```python
from build123d import *

# Parameters (mm, degrees)
SKETCH1_R           = 50
BOSS_EXTRUDE1_DEPTH = 150
SKETCH2_R           = 50
BOSS_EXTRUDE2_DEPTH = 150


with BuildPart() as part:
    # Sketch1 → Boss-Extrude1 (new, symmetric)
    with BuildSketch(Plane(origin=(0, 0, 0), x_dir=(1, 0, 0), z_dir=(0, 1, 0))):
        with Locations(Location((0, 0, 0), (0, 0, 270))):
            Circle(SKETCH1_R)
    extrude(amount=BOSS_EXTRUDE1_DEPTH, both=True)

    # Sketch2 → Boss-Extrude2 (add, symmetric)
    with BuildSketch(Plane(origin=(0, 0, 0), x_dir=(0, 0, -1), z_dir=(1, 0, 0))):
        Circle(SKETCH2_R)
    extrude(amount=BOSS_EXTRUDE2_DEPTH, both=True)


solid = part.part
```
Check sheet for the modelled part. Datum: model origin and axes. Units: mm. A direction names the side the tool comes from. Give positions to 0.01 mm unless a question says otherwise; leave off trailing zeros. Order: outer loops, then holes, each group sorted by start corner. A loop starts at its lowest first (then second) coordinate and runs counter-clockwise, first axis right, second up. Notation, with made-up numbers: M -37.5,88.25 L 5.5,88.25 A8 cw 5.5,93.25 Z; hole C 89,-9 d7. An arc over 180 degrees is marked long. Answer in a Markdown table with one row per item.
1) Cross-section at D-D, the plane z = -21. Enter the section's corners in (x, y), plus the area to 3 significant figures.
Filled sheet:
| item | result |
|---|---|
| outline | M -150,-45.38 L -45.38,-45.38 L -45.38,-150 L 45.38,-150 L 45.38,-45.38 L 150,-45.38 L 150,45.38 L 45.38,45.38 L 45.38,150 L -45.38,150 L -45.38,45.38 L -150,45.38 Z |
| area | 46,200 mm2 |
2) Access from +Z, -Z, +X, -X, +Y, -Y to the whole of each face (thin tool, end or side, straight path). Record for faces 1 (the cylindrical face through (49.575, 92.717, -6.509)), 2 (the cylindrical face through (2.2, -90.62, -49.95)), 3 (the cylindrical face through (92.717, 49.575, 6.509)).
Filled sheet:
| item | result |
|---|---|
| face 1 | +Y |
| face 2 | -Y |
| face 3 | +X |
3) Thickness scan on L1, parallel to Z at x = 119, y = -1; L2, parallel to X at y = 96, z = 1.5; L3, parallel to X at y = -59.5, z = -6. Record the ranges inside material, lowest first. Write a range as [from, to].
Filled sheet:
| item | result |
|---|---|
| L1 | z = [-49.99, 49.99] |
| L2 | x = [-49.98, 49.98] |
| L3 | x = [-49.64, 49.64] |
4) Cross-section at C-C, the plane x = 15. Enter the section's corners in (y, z).
Filled sheet:
| item | result |
|---|---|
| outline | M -150,-47.7 L -15,-47.7 A50 ccw 15,-47.7 L 150,-47.7 L 150,47.7 L 15,47.7 A50 ccw -15,47.7 L -150,47.7 Z |
5) Gauge pin test, flat ends, axial feed: P1, Ø8, axis at x = 31, y = -32.5, coming from the +Z side; P2, Ø2, axis at x = -20, y = 19.5, coming from the -Z side; P3, Ø1.5, axis at x = 100, z = -36, coming from the -Y side. Record the tip position at first contact, or that the pin passes through.
Filled sheet:
| item | result |
|---|---|
| P1 | stops at z = 42.08 |
| P2 | stops at z = -46.45 |
| P3 | stops at y = -35.46 |
6) Cross-section at A-A, the plane z = 0. Enter the section's corners in (x, y), plus the area to 3 significant figures.
Filled sheet:
| item | result |
|---|---|
| outline | M -150,-50 L -50,-50 L -50,-150 L 50,-150 L 50,-50 L 150,-50 L 150,50 L 50,50 L 50,150 L -50,150 L -50,50 L -150,50 Z |
| area | 50,000 mm2 |
7) Cross-section at B-B, the plane y = -40. Enter the section's corners in (x, z), plus the area to 3 significant figures.
Filled sheet:
| item | result |
|---|---|
| outline | M -150,-30 L -40,-30 A50 ccw 40,-30 L 150,-30 L 150,30 L 40,30 A50 ccw -40,30 L -150,30 Z |
| area | 20,200 mm2 |
